Geometry: final body of the model. Coordinates: model frame, mm. A direction names the side the tool comes from. Round coordinates to 2 decimals unless told otherwise and drop trailing zeros. Order: outer loops, then holes, each group sorted by start corner. A loop starts at its lowest first (then second) coordinate and runs counter-clockwise, first axis right, second up. Notation, with made-up numbers: M 47,4 L 58,4 A18 ccw 58,38 Z; hole C 55.5,-29 d2. An arc over 180 degrees is marked long. Return JSON: item names as keys, results as strings. Group by question number.
Q1. Mould query, pull axis X, two halves, no side actions, for faces 1 (the face through (32, -35, 10)), 2 (the face through (50, 5, 10)), 3 (the face through (25, -26, 10)). Classes: released by +X, released by -X, zero draft, split by the parting line, or undercut.
Q2. Ray query, probe 1 along Z at (x, y) = (42.5, 7); probe 2 along Y at (x, z) = (21, 23); probe 3 along Z at (x, y) = (24.5, 18.5). Return the intervals inside material, ascending.
Q3. Cut plane C-C on y = 20. Output: boundary loops of the cut face in (x, z), and give its area (3 significant figures).
Q4. Cut plane B-B on x = -22. Output: boundary loops of the cut face in (y, z), and give its area (3 significant figures).
Q5. Cut plane D-D on z = 38.5. Output: boundary loops of the cut face in (x, y), and give its area (3 significant figures).
Q6. Cut plane A-A on y = -21. Output: boundary loops of the cut face in (x, z).
Q7. Contact query for flat-ended pins moving along their axis: pin 1 (22 mm diameter, centred on x = 16.5, y = 26.5, fed in from +Z); pin 2 (10 mm diameter, centred on x = -12, z = 10, fed in from -Y); pin 3 (1 mm diameter, centred on x = 36.5, z = 56.5, fed in from +Y); pin 4 (1.5 mm diameter, centred on y = 23.5, z = 58.5, fed in from -X). Output: stop coordinate, or through.
Q8. Access query for faces 4 (the face through (-1, 35, 27)), 5 (the face through (-25, -26, 10)), 6 (the face through (-1, -4, 20)), 7 (the face through (-1, 25, 30)). Directions: +Z, -Z, +X, -X, +Y, -Y. A direction counts if a zero-diameter tool reaches every point of the face in a straight line with its end or side. Return the directions, or none.
```python
from build123d import *

# Parameters (mm, degrees)
EXTRUDE_1_DEPTH = 20
EXTRUDE_2_DEPTH = 20


with BuildPart() as part:
    # 草圖1 → 填料-伸長1 (new body)
    with BuildSketch(Plane.XY):
        with BuildLine():
            Line((25, -35), (40, -35))
            ThreePointArc((40, -35), (47.071067812, -32.071067812), (50, -25))
            Line((50, -25), (50, 35))
            Line((50, 35), (-50, 35))
            Line((-50, 35), (-50, -25))
            ThreePointArc((-50, -25), (-47.071067812, -32.071067812), (-40, -35))
            Line((-40, -35), (-25, -35))
            Line((-25, -35), (-25, -17.5))
            Line((-25, -17.5), (25, -17.5))
            Line((25, -17.5), (25, -35))
        make_face()
    extrude(amount=EXTRUDE_1_DEPTH)

    # 草圖2 → 填料-伸長2 (add)
    with BuildSketch(Plane(origin=(0, 35, 0), x_dir=(1, 0, 0), z_dir=(0, 1, 0))):
        with BuildLine():
            Line((50, -20), (-50, -20))
            ThreePointArc((-50, -20), (0, -70), (50, -20))
        make_face()
        with BuildLine():
            Line((-38.729833462, -30), (38.729833462, -30))
            ThreePointArc((38.729833462, -30), (0, -60), (-38.729833462, -30))
        make_face(mode=Mode.SUBTRACT)
    extrude(amount=-EXTRUDE_2_DEPTH)


solid = part.part
```
Result sheet:
{
 "1": {"face 1": "zero draft", "face 2": "released by +X", "face 3": "undercut"},
 "2": {"probe 1": "z = 0 to 20", "probe 2": "y = 15 to 35", "probe 3": "z = 0 to 30, 51.62 to 63.59"},
 "3": {"outline": "M -50,0 L 50,0 L 50,20 A50 ccw -50,20 Z; hole M -38.73,30 L 38.73,30 A40 ccw Z", "area": "4,210 mm²"},
 "4": {"outline": "M -17.5,0 L 35,0 L 35,30 L 15,30 L 15,20 L -17.5,20 Z; M 15,53.41 L 35,53.41 L 35,64.9 L 15,64.9 Z", "area": "1,480 mm²"},
 "5": {"outline": "M -46.45,15 L -35.46,15 L -35.46,35 L -46.45,35 Z; M 35.46,15 L 46.45,15 L 46.45,35 L 35.46,35 Z", "area": "439 mm²"},
 "6": {"outline": "M -50,0 L -25,0 L -25,20 L -50,20 Z; M 25,0 L 50,0 L 50,20 L 25,20 Z"},
 "7": {"pin 1": "stops at z = 69.7", "pin 2": "stops at y = -17.5", "pin 3": "passes through", "pin 4": "stops at x = -32.79"},
 "8": {"face 4": "+Z, -Z, +X, -X, +Y", "face 5": "+Z, -Z, -Y", "face 6": "+Z, +X, -X, -Y", "face 7": "+Y, -Y"}
}
